Geometry: final body of the model. Coordinates: model frame, mm. Face numbers are marked on the shaded views. A direction names the side the tool comes from. Give positions to 0.01 mm unless a question says otherwise; leave off trailing zeros. Loops run counter-clockwise (first coordinate to the right, second up) from the corner with the lowest first, then second, coordinate; pieces in that order, holes last. Notation, with made-up numbers: (13.5, 55.5) -> (20.5, 55.5) arc R27 ccw to (20.5, 90.5) -> close; hole circle Ø5 at (-18.75, 40.5). An arc over 180 degrees is marked (long way). Answer in a Markdown table with one row per item. Add a question column.
1) Line query: line 1 (X direction, y = -3.75, z = 0); line 2 (X direction, y = -9.7, z = 0); line 3 (Z direction, x = 0.25, y = -10.75). Output: solid intervals per line, ascending. Write a range as from..to.
2) Section query B-B (z = 0). Return the cut outline in (x, y).
3) Access query for the marked faces 5, 6 and 7. Directions: +Z, -Z, +X, -X, +Y, -Y. A direction counts if a zero-diameter tool reaches every point of the face in a straight line with its end or side. Return the directions, or none.
4) Section query A-A (x = 0). Return the cut outline in (y, z).
5) Section query C-C (y = -8.75). Return the cut outline in (x, z).
6) First-contact query: P1, Ø2, axis at x = 0, y = -5.5, coming from the +Z side; P2, Ø0.5, axis at y = -0.5, z = -2, coming from the -X side; P3, Ø1.8, axis at x = 0, z = 0, coming from the -Y side. Flat tips, straight axial feed; report the tip coordinate or a pass-through.
7) Draft query along X for the marked faces 1, 2, 3 and 4. Return one class per face: +X half, -X half, draft (parallel to the pull), parting line (faces both ways), or undercut.
8) Section query D-D (y = -3.25). Return the cut outline in (x, z).
```python
from build123d import *

# Parameters (mm, degrees)
CHANFREIN1_SIZE         = 0.5
ESQUISSE3_W             = 1.4
ESQUISSE3_H             = 6
ENL_V_MAT_EXTRU_1_DEPTH = 1.5
ENL_V_START             = -8
ESQUISSE4_OUTSIDE_W     = 11.274
ESQUISSE4_OUTSIDE_H     = 11.274
ESQUISSE4_OUTSIDE_W_2   = 3.2
ESQUISSE4_OUTSIDE_H_2   = 3.2
ENL_V_MAT_EXTRU_2_DEPTH = 7


with BuildPart() as part:
    # Esquisse2 → Révolution1 (revolve)
    with BuildSketch(Plane.XY, mode=Mode.PRIVATE) as r_volution1_sk:
        with BuildLine():
            Line((-0.8, 0), (-3, 0))
            Line((-3, 0), (-3, -2))
            Line((-3, -2), (-2, -3))
            Line((-2, -3), (-2, -13.82503854))
            ThreePointArc((-2, -13.82503854), (-1.60238974, -13.923446201), (-1.2, -14))
            Line((-1.2, -14), (-1.2, -8))
            Line((-1.2, -8), (-0.8, -8))
            Line((-0.8, -8), (-0.8, 0))
        make_face()
    revolve(r_volution1_sk.sketch.rotate(Axis((0, -17.325308642, 0), (0, 1, 0)), 270), axis=Axis((0, -17.325308642, 0), (0, 1, 0)))  # turned: the seam where the file's is

    # Chanfrein1
    chanfrein1_edges = [part.edges().sort_by_distance(p)[0] for p in [
        (0, 0, 3),
    ]]
    chamfer(chanfrein1_edges, length=CHANFREIN1_SIZE)

    # Esquisse3 → Enlèv. mat.-Extru.1 (cut)
    with BuildSketch(Plane(origin=(0, 0, 0), x_dir=(-1, 0, 0), z_dir=(0, 1, 0))):
        Rectangle(ESQUISSE3_W, ESQUISSE3_H)
    extrude(amount=-ENL_V_MAT_EXTRU_1_DEPTH, mode=Mode.SUBTRACT)

    # Esquisse4 outside → Enlèv. mat.-Extru.2 (cut, through all)
    with BuildSketch(Plane(origin=(0, 0, 0), x_dir=(-1, 0, 0), z_dir=(0, 1, 0)).offset(ENL_V_START)):
        Rectangle(ESQUISSE4_OUTSIDE_W, ESQUISSE4_OUTSIDE_H)
        Rectangle(ESQUISSE4_OUTSIDE_W_2, ESQUISSE4_OUTSIDE_H_2, mode=Mode.SUBTRACT)
    extrude(amount=-ENL_V_MAT_EXTRU_2_DEPTH, mode=Mode.SUBTRACT)


solid = part.part
```
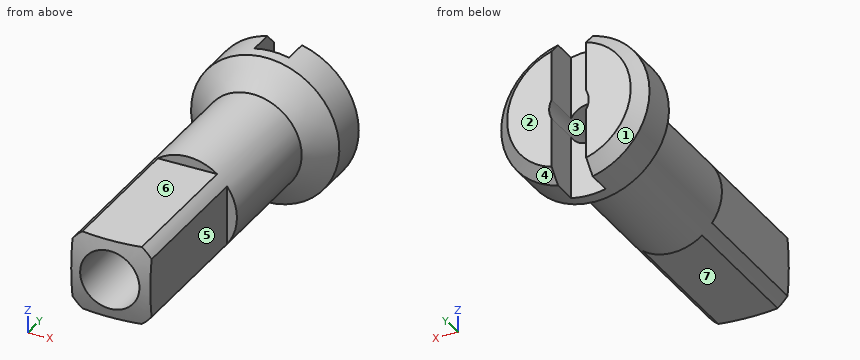
Evaluation:
| question | item | result |
|---|---|---|
| 1 | line 1 | -2..-0.8, 0.8..2 |
| 1 | line 2 | -1.6..-1.2, 1.2..1.6 |
| 1 | line 3 | -1.6..-1.17, 1.17..1.6 |
| 2 | outline | (-3, -2) -> (-2, -3) -> (-2, -8) -> (-1.6, -8) -> (-1.6, -13.92) arc R7.5 ccw to (-1.2, -14) -> (-1.2, -8) -> (-0.8, -8) -> (-0.8, 0) -> (-2.5, 0) -> (-3, -0.5) -> close; (0.8, -8) -> (1.2, -8) -> (1.2, -14) arc R7.5 ccw to (1.6, -13.92) -> (1.6, -8) -> (2, -8) -> (2, -3) -> (3, -2) -> (3, -0.5) -> (2.5, 0) -> (0.8, 0) -> close |
| 3 | face 5 | +Z, -Z, +X, -Y |
| 3 | face 6 | +Z, +X, -X, -Y |
| 3 | face 7 | -Z, +X, -X, -Y |
| 4 | outline | (-14, -1.2) arc R7.5 ccw to (-13.92, -1.6) -> (-8, -1.6) -> (-8, -2) -> (-3, -2) -> (-2, -3) -> (-1.5, -3) -> (-1.5, -0.8) -> (-8, -0.8) -> (-8, -1.2) -> close; (-14, 1.2) -> (-8, 1.2) -> (-8, 0.8) -> (-1.5, 0.8) -> (-1.5, 3) -> (-2, 3) -> (-3, 2) -> (-8, 2) -> (-8, 1.6) -> (-13.92, 1.6) arc R7.5 ccw to start |
| 5 | outline | (-1.6, -1.2) arc R2 ccw to (-1.2, -1.6) -> (1.2, -1.6) arc R2 ccw to (1.6, -1.2) -> (1.6, 1.2) arc R2 ccw to (1.2, 1.6) -> (-1.2, 1.6) arc R2 ccw to (-1.6, 1.2) -> close; hole circle Ø2.4 at (0, 0) |
| 6 | P1 | z = 2 |
| 6 | P2 | x = -2.44 |
| 6 | P3 | y = -8 |
| 7 | face 1 | -X half |
| 7 | face 2 | draft |
| 7 | face 3 | undercut |
| 7 | face 4 | +X half |
| 8 | outline | circle Ø4 at (0, 0); hole circle Ø1.6 at (0, 0) |
